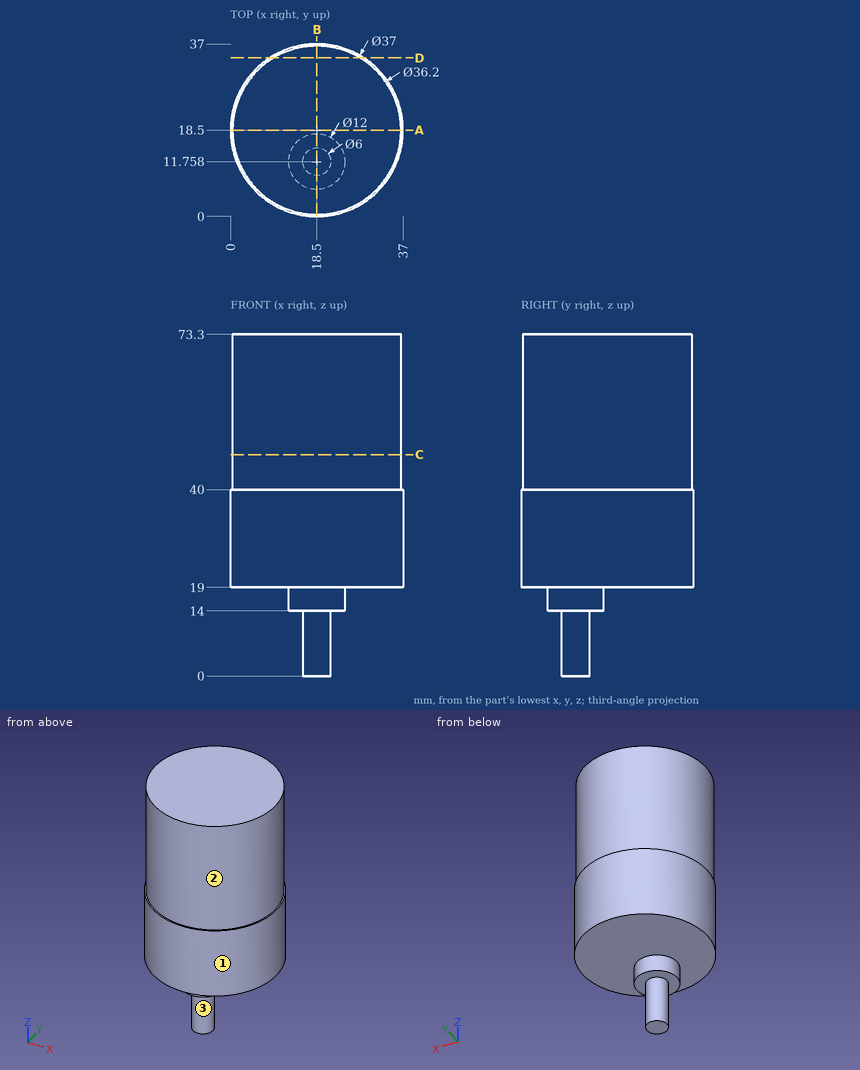
Can you work these out from the drawing? Everything is in mm from the part's minimum corner. A direction names the side the tool comes from. Round coordinates to 2 decimals unless told otherwise and drop trailing zeros. Loops run counter-clockwise (first coordinate to the right, second up) from the corner with the lowest first, then second, coordinate; pieces in that order, holes last. Notation, with made-up numbers: (12, 76.25) -> (44, 76.25) arc R23 ccw to (44, 89.25) -> close; hole circle Ø7 at (61, 69). An arc over 180 degrees is marked (long way). Use CSV: the item, a comma, the result in double quotes.
(1) Suppose I cut it at B-B on x = 18.5. Write out the boundary of the cut face in (y, z).
Return value:
outline,"(0, 19) -> (5.76, 19) -> (5.76, 14) -> (8.76, 14) -> (8.76, 0) -> (14.76, 0) -> (14.76, 14) -> (17.76, 14) -> (17.76, 19) -> (37, 19) -> (37, 40) -> (36.6, 40) -> (36.6, 73.3) -> (0.4, 73.3) -> (0.4, 40) -> (0, 40) -> close"
(2) For the marked faces 1, 2 and 3, which set-ups out of +Z, -Z, +X, -X, +Y, -Y let a thin tool reach every point of the face, with its end or its side?
Return value:
face 1,"+Z, -Z"
face 2,"+Z"
face 3,"-Z"
(3) Suppose I cut it at C-C on z = 47.5. Write out the boundary of the cut face in (x, y), plus the area to 3 significant figures.
Return value:
outline,"circle Ø36.2 at (18.5, 18.5)"
area,"1,030 mm²"
(4) Suppose I cut it at D-D on y = 34. Write out the boundary of the cut face in (x, z).
Return value:
outline,"(8.4, 19) -> (28.6, 19) -> (28.6, 40) -> (27.85, 40) -> (27.85, 73.3) -> (9.15, 73.3) -> (9.15, 40) -> (8.4, 40) -> close"
(5) Suppose I cut it at A-A on y = 18.5. Write out the boundary of the cut face in (x, z).
Return value:
outline,"(0, 19) -> (37, 19) -> (37, 40) -> (36.6, 40) -> (36.6, 73.3) -> (0.4, 73.3) -> (0.4, 40) -> (0, 40) -> close"
(6) Will these pins go through, and if not, where does the flat tip stop? pin 1 Ø1.5 at (y, z) = (29, 34.5) entering from +X; pin 2 Ø12 at (x, y) = (19.5, 33) entering from -Z; pin 3 Ø8 at (x, z) = (5.5, 44) entering from +Y.
Return value:
pin 1,"stops at x = 34.22"
pin 2,"stops at z = 19"
pin 3,"stops at y = 34.2"
(7) If I drill on probe 1 along Z at (x, y) = (3, 17); probe 2 along Z at (x, y) = (18, 7); probe 3 along X at (y, z) = (18, 20), over which ranges is the centre line in solid material (lowest first)? Write a range as [from, to].
Return value:
probe 1,"z = [19, 73.3]"
probe 2,"z = [14, 73.3]"
probe 3,"x = [0.01, 36.99]"
